Work out the finished part from the listing and answer in its coordinate system (mm). A direction names the side the tool comes from. Round coordinates to 2 decimals unless told otherwise and drop trailing zeros. Loops run counter-clockwise (first coordinate to the right, second up) from the corner with the lowest first, then second, coordinate; pieces in that order, holes last.
Autodesk Inventor part; units mm, degrees
ref_plane "YZ Plane" through (0, 0, 0) normal (1, 0, 0) x (0, 1, 0)
ref_plane "XZ Plane" through (0, 0, 0) normal (0, 1, 0) x (-1, 0, 0)
ref_plane "XY Plane" through (0, 0, 0) normal (0, 0, 1) x (1, 0, 0)
sketch "Эскиз1" plane through (0, 0, 0) normal (0, 1, 0) x (-1, 0, 0)
  circle A0 centre (0, 0) radius 2.25
  circle A1 centre (0, 0) radius 2.75
  circle A2 centre (0, 0) radius 3.5
  dimension "d0" = 4.5
  dimension "d1" = 5.5
  dimension "d2" = 7
extrude "Выдавливание1" add sketch "Эскиз1" against normal blind 4 contours A0 | A1 | A2
extrude "Выдавливание2" add sketch "Эскиз1" against normal blind 15 contours A0
extrude "Выдавливание3" add sketch "Эскиз1" along normal blind 7 contours A2
chamfer "Фаска1" distance 0.5 angle 45 3 edges at (3.5, -4, 0) (2.25, -15, 0) (2.75, 7, 0)
properties part number "connector"
1. Which of the six approach directions +Z, -Z, +X, -X, +Y, -Y give full straight-line access (tool end or side, diameter ignored) to faces 1 (the face through (-3.233, 1.824, -1.341)), 2 (the face through (0.596, 3.204, 2.685))?
Answer key:
face 1: +Y, -Y
face 2: +Y
2. Given pin 1 (1 mm diameter, centred on x = -1.5, y = 4, fed in from -Z); pin 2 (1 mm diameter, centred on y = 2, z = 2.5, fed in from +X); pin 3 (1 mm diameter, centred on x = 2, y = -2, fed in from -Z), each flat-ended and moving along its own axis, determine where each tip first touches the part or whether it passes through.
Answer key:
pin 1: stops at z = -3.35
pin 2: stops at x = 2.87
pin 3: stops at z = -3.16
3. Find section B-B (x = 0). Write down the section's boundary in (y, z).
Answer key:
outline: (-15, -1.75) - (-14.5, -2.25) - (-4, -2.25) - (-4, -3) - (-3.5, -3.5) - (7, -3.5) - (7, -3.25) - (6.5, -2.75) - (0, -2.75) - (0, 2.75) - (6.5, 2.75) - (7, 3.25) - (7, 3.5) - (-3.5, 3.5) - (-4, 3) - (-4, 2.25) - (-14.5, 2.25) - (-15, 1.75) - close
4. Find section A-A (z = 0). Write down the section's boundary in (x, y), then the cut area to 4 significant figures.
Answer key:
outline: (-3.5, -3.5) - (-3, -4) - (-2.25, -4) - (-2.25, -14.5) - (-1.75, -15) - (1.75, -15) - (2.25, -14.5) - (2.25, -4) - (3, -4) - (3.5, -3.5) - (3.5, 7) - (3.25, 7) - (2.75, 6.5) - (2.75, 0) - (-2.75, 0) - (-2.75, 6.5) - (-3.25, 7) - (-3.5, 7) - close
area: 87.25 mm2
5. Find section D-D (y = -11). Write down the section's boundary in (x, z), then the cut area to 3 significant figures.
Answer key:
outline: circle Ø4.5 at (0, 0)
area: 15.9 mm2
6. Find section C-C (y = 4.25). Write down the section's boundary in (x, z).
Answer key:
outline: circle Ø7 at (0, 0); hole circle Ø5.5 at (0, 0)
7. Determine the mould class of faces 3 (the face through (0, -15, 0)), 4 (the face through (0, 0, 0)), 5 (the face through (0.29, -9.18, 2.23)) for opening direction Z: +Z half, -Z half, draft (parallel to the pull), parting line (faces both ways), or undercut.
Answer key:
face 3: draft
face 4: undercut
face 5: parting line
8. Consider probe 1 along Z at (x, y) = (0, 2); probe 2 along Y at (x, z) = (0.25, 1.5); probe 3 along Y at (x, z) = (-2, 1.25). Determine where each line is inside the solid, lowest interval first.
Answer key:
probe 1: z = -3.5 to -2.75, 2.75 to 3.5
probe 2: y = -15 to 0
probe 3: y = -4 to 0
